For this review, take the finished solid that the model builds, in its own axes (mm). Face numbers are marked on the shaded views. Round coordinates to 2 decimals unless told otherwise and drop trailing zeros. Order: outer loops, then holes, each group sorted by start corner. A loop starts at its lowest first (then second) coordinate and runs counter-clockwise, first axis right, second up. Notation, with made-up numbers: (88.5, 24) -> (145.5, 24) arc R16 cw to (145.5, 52) -> close; hole circle Ø10 at (65.5, -15). An arc over 180 degrees is marked (long way). Answer in a Markdown table with one row per item.
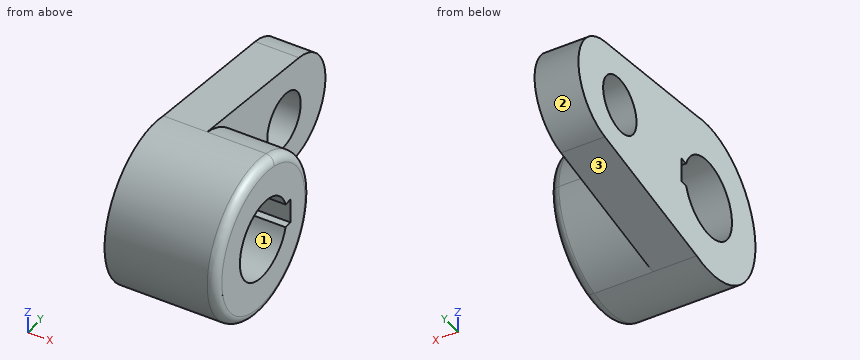
```python
from build123d import *

# Parameters (mm, degrees)
F1_DEPTH = 40.2336
F0_R     = 10.16
F2_DEPTH = 15.7734
F3_R     = 3.302


with BuildPart() as f1:
    # F0 (on Right) → F1 (new body)
    with BuildSketch(Plane.YZ):
        with BuildLine():
            ThreePointArc((7.18307, -27.657443), (22.602952, -17.482483), (28.575, 0))
            ThreePointArc((28.575, 0), (22.602952, 17.482483), (7.18307, 27.657443))
            ThreePointArc((7.18307, 27.657443), (-28.575, 0), (7.18307, -27.657443))
        make_face()
        with BuildLine():
            ThreePointArc((13.559429, -4.502727), (-14.2875, 0), (13.559429, 4.502727))
            Line((13.559429, 4.502727), (16.4084, 4.502727))
            Line((16.4084, 4.502727), (16.4084, -4.502727))
            Line((16.4084, -4.502727), (13.559429, -4.502727))
        make_face(mode=Mode.SUBTRACT)
    extrude(amount=F1_DEPTH)

    # F0 (on Right) → F2 (join)
    with BuildSketch(Plane.YZ):
        with BuildLine():
            ThreePointArc((7.18307, -27.657443), (22.602952, -17.482483), (28.575, 0))
            ThreePointArc((28.575, 0), (22.602952, 17.482483), (7.18307, 27.657443))
            ThreePointArc((7.18307, 27.657443), (-28.575, 0), (7.18307, -27.657443))
        make_face()
        with BuildLine():
            ThreePointArc((13.559429, -4.502727), (-14.2875, 0), (13.559429, 4.502727))
            Line((13.559429, 4.502727), (16.4084, 4.502727))
            Line((16.4084, 4.502727), (16.4084, -4.502727))
            Line((16.4084, -4.502727), (13.559429, -4.502727))
        make_face(mode=Mode.SUBTRACT)
        with BuildLine():
            ThreePointArc((7.18307, 27.657443), (22.602952, 17.482483), (28.575, 0))
            ThreePointArc((28.575, 0), (22.602952, -17.482483), (7.18307, -27.657443))
            Line((7.18307, -27.657443), (63.100665, -18.816257))
            ThreePointArc((63.100665, -18.816257), (79.175608, 0), (63.100665, 18.816257))
            Line((63.100665, 18.816257), (7.18307, 27.657443))
        make_face()
        with Locations((53.975, 0)):
            Circle(F0_R, mode=Mode.SUBTRACT)
    extrude(amount=F2_DEPTH)

    # F3
    f3_edges = [f1.edges().sort_by_distance(p)[0] for p in [
        (40.2336, -7.18307, 27.657443),
    ]]
    fillet(f3_edges, radius=F3_R)


solid = f1.part
```
Q1. The part is to be moulded in two halves that separate along Z. For the marked faces 1, 2 and 3, say which applies: +Z half, -Z half, draft (parallel to the pull), parting line (faces both ways), or undercut.
Answer key:
| item | result |
|---|---|
| face 1 | undercut |
| face 2 | parting line |
| face 3 | -Z half |
Q2. To check wall thickness, follow probe 1 along Z at (x, y) = (23.5, 0.5); probe 2 along X at (y, z) = (34, 8); probe 3 along Y at (x, z) = (25, 6.5). State the ranges of each line that lie inside material, in increasing order.
Answer key:
| item | result |
|---|---|
| probe 1 | z = -28.57 to -14.28, 14.28 to 28.57 |
| probe 2 | x = 0 to 15.77 |
| probe 3 | y = -27.83 to -12.72, 12.72 to 27.83 |
Q3. Clearance check with flat-ended pins moving along their axes: pin 1 Ø12 at (x, y) = (11, -11) entering from -Z; pin 2 Ø10 at (x, z) = (18.5, 1.5) entering from -Y (3 decimals); pin 3 Ø2 at (x, z) = (33.5, 16.5) entering from -Y; pin 4 Ø2 at (x, z) = (28, 14.5) entering from -Y. State where each tip first meets the part, or that it passes through.
Answer key:
| item | result |
|---|---|
| pin 1 | stops at z = -28.13 |
| pin 2 | stops at y = -28.575 |
| pin 3 | stops at y = -24.01 |
| pin 4 | stops at y = -25.18 |
Q4. Take a section at A-A, the plane x = 14.5. Give the number of separate pieces and of enclosed holes in the cut face, then the cut area to 3 significant figures.
Answer key:
| item | result |
|---|---|
| separate pieces | 1 |
| enclosed holes | 2 |
| area | 3,760 mm^2 |
Q5. Take a section at D-D, the plane y = 32. Write out the cut boundary in (x, z).
Answer key:
| item | result |
|---|---|
| outline | (0, -23.73) -> (15.77, -23.73) -> (15.77, 23.73) -> (0, 23.73) -> close |
